```python
from build123d import *

# Parameters (mm, degrees)
EXTRUDE_1_DEPTH          = 10
CUT_EXTRUDE_1_DEPTH      = 112.11599651
CUT_EXTRUDE_1_DEPTH_BACK = 5
SKETCH_2_R               = 8.120196397
SKETCH_3_R               = 2.466762855
CUT_EXTRUDE_2_DEPTH      = 5


with BuildPart() as part:
    # 草图1 → 凸台-拉伸1 (new body)
    with BuildSketch(Plane.XY):
        with BuildLine():
            Line((13.670219887, 7.404471095), (102.163149927, 7.404471095))
            ThreePointArc((102.163149927, 7.404471095), (109.567621023, 0), (102.163149927, -7.404471095))
            Line((102.163149927, -7.404471095), (13.670219887, -7.404471095))
            ThreePointArc((13.670219887, -7.404471095), (-15.546739336, 0), (13.670219887, 7.404471095))
        make_face()
    extrude(amount=EXTRUDE_1_DEPTH)

    # 草图2 → 切除-拉伸1 (cut, two sides: drawn at the far end of the back side and taken through both)
    with BuildSketch(Plane(origin=(0, 0, 0), x_dir=(-1, 0, 0), z_dir=(0, 0, -1)).offset(-CUT_EXTRUDE_1_DEPTH_BACK)):
        with Locations(Location((0, 0, 0), (0, 0, 180))):
            Circle(SKETCH_2_R)
    extrude(amount=CUT_EXTRUDE_1_DEPTH + CUT_EXTRUDE_1_DEPTH_BACK, mode=Mode.SUBTRACT)

    # 草图3 → 切除-拉伸2 (cut)
    with BuildSketch(Plane.XY.offset(10)):
        Circle(SKETCH_3_R)
    extrude(amount=-CUT_EXTRUDE_2_DEPTH, mode=Mode.SUBTRACT)


solid = part.part
```
Verification items for the finished model (mm, model axes). A direction names the side the tool comes from. Give positions to 0.01 mm unless a question says otherwise; leave off trailing zeros. Loops run counter-clockwise (first coordinate to the right, second up) from the corner with the lowest first, then second, coordinate; pieces in that order, holes last.
1. Set-up check for faces 1 (the flat face through (48, 0, 0)), 2 (the flat face through (59, -7.404, 5)), 3 (the flat face through (2, -2, 5)): record each of +Z, -Z, +X, -X, +Y, -Y from which the full face is reachable in a straight line by a thin tool's end or side.
2. Thickness scan on line 1 (Y direction, x = 0, z = 7.05); line 2 (Y direction, x = 98.5, z = 9); line 3 (Y direction, x = 0, z = 3.9). Record the ranges inside material, lowest first.
3. Section check B-B, the plane y = 0. Enter the section's corners in (x, z), then the cut area to 3 significant figures.
4. Section check D-D, the plane x = 80.5. Enter the section's corners in (y, z), then the cut area to 3 significant figures.
5. Mould release check, pull along X, two halves, no side actions. Record for faces 4 (the cylindrical face through (-0.53, -2.41, 7.54)), 5 (the cylindrical face through (-15.536, -0.576, 4.93)), 6 (the flat face through (57, 7.404, 5)): released by +X, released by -X, zero draft, split by the parting line, or undercut.
6. Section check C-C, the plane z = 2.75. Enter the section's corners in (x, y), then the cut area to 3 significant figures.
7. Section check A-A, the plane x = 0. Enter the section's corners in (y, z).
8. Go/stop test with flat-tipped pins: pin 1 Ø5 at (x, y) = (91, 11) entering from +Z; pin 2 Ø1.5 at (x, y) = (62.5, -0.5) entering from -Z; pin 3 Ø1.5 at (x, z) = (48.5, 4) entering from +Y; pin 4 Ø1 at (y, z) = (7, 1) entering from +X. Record where each tip stops, or that it passes through.
Geometry says:
1. face 1: -Z, +X, -X, +Y, -Y
1. face 2: +Z, -Z, +X, -Y
1. face 3: -Z
2. line 1: y = -15.55 to -2.47, 2.47 to 15.55
2. line 2: y = -7.4 to 7.4
2. line 3: y = -15.55 to -8.12, 8.12 to 15.55
3. outline: (-15.55, 0) - (-8.12, 0) - (-8.12, 5) - (-2.47, 5) - (-2.47, 10) - (-15.55, 10) - close; (2.47, 5) - (8.12, 5) - (8.12, 0) - (109.57, 0) - (109.57, 10) - (2.47, 10) - close
3. area: 1,150 mm2
4. outline: (-7.4, 0) - (7.4, 0) - (7.4, 10) - (-7.4, 10) - close
4. area: 148 mm2
5. face 4: undercut
5. face 5: split by the parting line
5. face 6: zero draft
6. outline: (13.67, -7.4) - (102.16, -7.4) arc R7.4 ccw to (102.16, 7.4) - (13.67, 7.4) arc R15.55 ccw (long way) to start; hole circle Ø16.24 at (0, 0)
6. area: 1,930 mm2
7. outline: (-15.55, 0) - (-8.12, 0) - (-8.12, 5) - (-2.47, 5) - (-2.47, 10) - (-15.55, 10) - close; (2.47, 5) - (8.12, 5) - (8.12, 0) - (15.55, 0) - (15.55, 10) - (2.47, 10) - close
8. pin 1: passes through
8. pin 2: stops at z = 0
8. pin 3: stops at y = 7.4
8. pin 4: stops at x = 105.71
